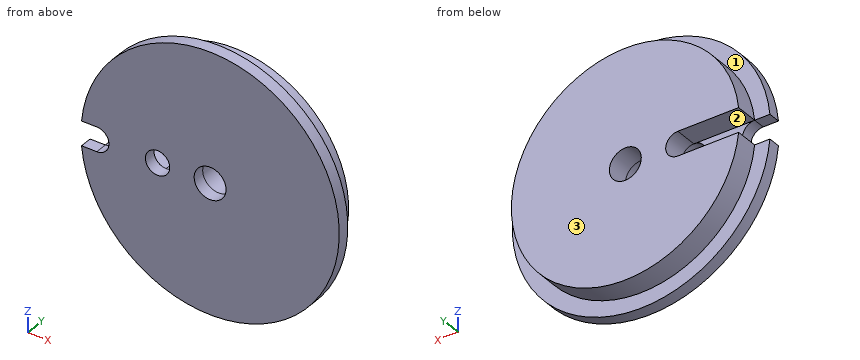
```python
from build123d import *

# Parameters (mm, degrees)
SKETCH_1_R          = 15
SKETCH_1_R_2        = 2.1
EXTRUDE_1_DEPTH     = 3
CUT_EXTRUDE_1_DEPTH = 10
SKETCH_3_R          = 1.6
SKETCH_3_R_2        = 2.1
EXTRUDE_2_DEPTH     = 1.6


with BuildPart() as part:
    # ｽｹｯﾁ1 → ﾎﾞｽ - 押し出し1 (new body)
    with BuildSketch(Plane(origin=(0, 0, 0), x_dir=(1, 0, 0), z_dir=(0, 1, 0))):
        with Locations(Location((0, 0, 0), (0, 0, 270))):
            Circle(SKETCH_1_R)
        with Locations(Location((0, 0, 0), (0, 0, 270))):
            Circle(SKETCH_1_R_2, mode=Mode.SUBTRACT)
    extrude(amount=EXTRUDE_1_DEPTH)

    # ｽｹｯﾁ2 → ｶｯﾄ - 押し出し1 (cut)
    with BuildSketch(Plane(origin=(0, 3, 0), x_dir=(1, 0, 0), z_dir=(0, 1, 0))):
        with BuildLine():
            Line((-14.91442255, 1.6), (-6.91442255, 1.6))
            ThreePointArc((-6.91442255, 1.6), (-5.31442255, 0), (-6.91442255, -1.6))
            Line((-6.91442255, -1.6), (-14.91442255, -1.6))
            ThreePointArc((-14.91442255, -1.6), (-16.51442255, 0), (-14.91442255, 1.6))
        make_face()
    extrude(amount=-CUT_EXTRUDE_1_DEPTH, mode=Mode.SUBTRACT)

    # ｽｹｯﾁ3 → ﾎﾞｽ - 押し出し2 (add)
    with BuildSketch(Plane.XZ):
        with BuildLine():
            Line((-16.924538398, -1.6), (-14.91442255, -1.6))
            ThreePointArc((-14.91442255, -1.6), (-13.31442255, 0), (-14.91442255, 1.6))
            Line((-14.91442255, 1.6), (-16.924538398, 1.6))
            ThreePointArc((-16.924538398, 1.6), (17, 0), (-16.924538398, -1.6))
        make_face()
        with Locations(Location((-6.91442255, 0, 0), (0, 0, 270))):
            Circle(SKETCH_3_R, mode=Mode.SUBTRACT)
        with Locations(Location((0, 0, 0), (0, 0, 270))):
            Circle(SKETCH_3_R_2, mode=Mode.SUBTRACT)
    extrude(amount=EXTRUDE_2_DEPTH)


solid = part.part
```
The model under review builds one solid part; all positions refer to its coordinate system, in mm. Face numbers are marked on the shaded views. A direction names the side the tool comes from. Round coordinates to 2 decimals unless told otherwise and drop trailing zeros. Loops run counter-clockwise (first coordinate to the right, second up) from the corner with the lowest first, then second, coordinate; pieces in that order, holes last. Notation, with made-up numbers: M 15.25,33 L 71.25,33 A9 cw 71.25,45 Z; hole C 35,-38.5 d5. An arc over 180 degrees is marked long. Answer as a JSON object with one key per item and string values.
(1) Take a section at B-B on x = 0. Give the boundary of the cut face in (y, z).
Resolved:
{"outline": "M -1.6,-17 L 0,-17 L 0,-15 L 3,-15 L 3,-2.1 L -1.6,-2.1 Z; M -1.6,2.1 L 3,2.1 L 3,15 L 0,15 L 0,17 L -1.6,17 Z"}
(2) Take a section at D-D on y = -0.5. Give the boundary of the cut face in (x, z), and give its area (3 significant figures).
Resolved:
{"outline": "M -16.92,-1.6 A17 ccw long -16.92,1.6 L -14.91,1.6 A1.6 cw -14.91,-1.6 Z; hole C -6.91,0 d3.2; hole C 0,0 d4.2", "area": "875 mm²"}
(3) Take a section at C-C on y = 2.3. Give the boundary of the cut face in (x, z), and give its area (3 significant figures).
Resolved:
{"outline": "M -14.91,-1.6 A15 ccw long -14.91,1.6 L -6.91,1.6 A1.6 cw -6.91,-1.6 Z; hole C 0,0 d4.2", "area": "663 mm²"}
(4) Take a section at A-A on z = 0. Give the boundary of the cut face in (x, y).
Resolved:
{"outline": "M -13.31,-1.6 L -8.51,-1.6 L -8.51,0 L -13.31,0 Z; M -5.31,-1.6 L -2.1,-1.6 L -2.1,3 L -5.31,3 Z; M 2.1,-1.6 L 17,-1.6 L 17,0 L 15,0 L 15,3 L 2.1,3 Z"}
(5) To check wall thickness, follow line 1 along X through (y, z) = (-1.3, 0); line 2 along Z through (x, y) = (0, -0.5); line 3 along Z through (x, y) = (0, 0.85). State the ranges of each line that lie inside material, in increasing order.
Resolved:
{"line 1": "-13.31 to -8.51, -5.31 to -2.1, 2.1 to 17", "line 2": "-17 to -2.1, 2.1 to 17", "line 3": "-15 to -2.1, 2.1 to 15"}
(6) Tool access review of the marked faces 1, 2 and 3: name each direction out of +Z, -Z, +X, -X, +Y, -Y from which nothing blocks a thin tool from reaching the whole face with its end or side.
Resolved:
{"face 1": "+Y", "face 2": "-X, +Y", "face 3": "+Z, -Z, +X, -X, +Y"}
(7) Clearance check with flat-ended pins moving along their axes: P1, Ø1, axis at x = -10.5, z = 0.5, coming from the +Y side; P2, Ø2.5, axis at x = -10, y = 2, coming from the +Z side; P3, Ø0.5, axis at x = -16, y = -0.5, coming from the -Z side. State where each tip first meets the part, or that it passes through.
Resolved:
{"P1": "y = 0", "P2": "z = 12.18", "P3": "z = -6.4"}
